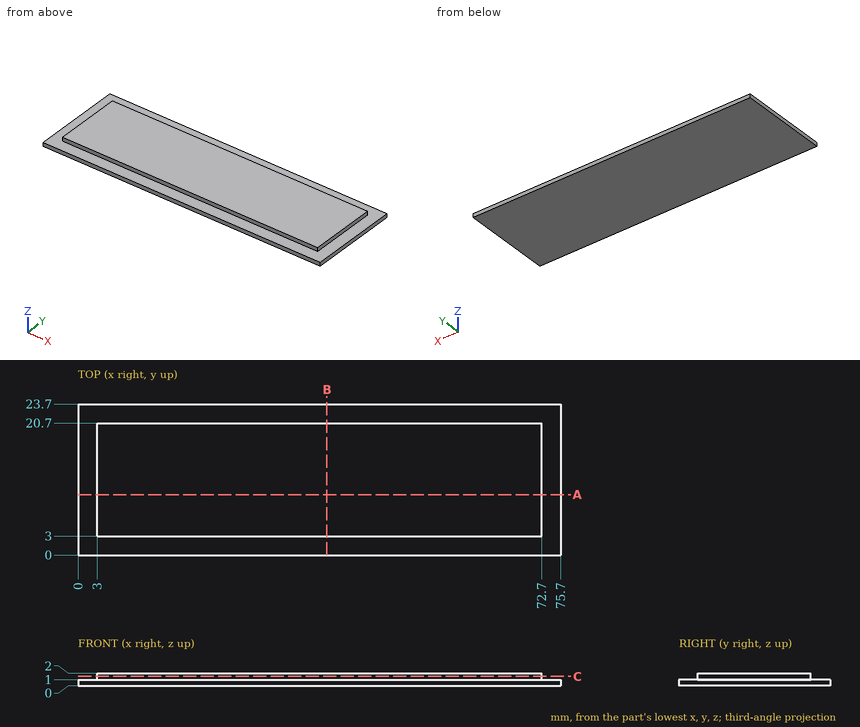
Part print with two shaded views. Sizes in mm from the minimum x, y, z corner. Coordinates: 2 decimals unless noted, no trailing zeros. Loops run counter-clockwise (first coordinate to the right, second up) from the corner with the lowest first, then second, coordinate; pieces in that order, holes last. Notation, with made-up numbers: M -35,53.25 L 17,53.25 A5 cw 17,59.25 Z; hole C -18.5,55.5 d4. An arc over 180 degrees is marked long. Use CSV: the item, a comma, the result in double quotes. Start each with the question number.
1. Flat gauge pins, fed straight in: pin 1 (0.8 mm diameter, centred on y = 10, z = 1.5, fed in from +X); pin 2 (0.5 mm diameter, centred on y = 13.5, z = 1.5, fed in from -X). Where does each tip first touch, or does it go through?
2. Band-saw the part on B-B, the plane x = 39. List the corners of the cut face in (y, z), then the cut area to 3 significant figures.
3. Band-saw the part on C-C, the plane z = 1.5. List the corners of the cut face in (x, y).
4. Band-saw the part on A-A, the plane y = 9.5. List the corners of the cut face in (x, z).
5. Probe probe 1 along X at (y, z) = (17.25, 1.2); probe 2 along Z at (x, y) = (14.5, 2.75); probe 3 along Y at (x, z) = (45.5, 1.9). List the from-to ranges inside material, lowest first. Write a range as [from, to].
Entries:
1,pin 1,"stops at x = 72.7"
1,pin 2,"stops at x = 3"
2,outline,"M 0,0 L 23.7,0 L 23.7,1 L 20.7,1 L 20.7,2 L 3,2 L 3,1 L 0,1 Z"
2,area,"41.4 mm2"
3,outline,"M 3,3 L 72.7,3 L 72.7,20.7 L 3,20.7 Z"
4,outline,"M 0,0 L 75.7,0 L 75.7,1 L 72.7,1 L 72.7,2 L 3,2 L 3,1 L 0,1 Z"
5,probe 1,"x = [3, 72.7]"
5,probe 2,"z = [0, 1]"
5,probe 3,"y = [3, 20.7]"
